from build123d import *

# Parameters (mm, degrees)
CROQUIS2_W              = 140
CROQUIS2_H              = 140
CROQUIS2_R              = 1.5
CROQUIS2_R_2            = 6
CROQUIS2_W_2            = 40
CROQUIS2_H_2            = 5
CROQUIS2_W_3            = 5
CROQUIS2_H_3            = 40
SALIENTE_EXTRUIR1_DEPTH = 5


with BuildPart() as part:
    # Croquis2 → Saliente-Extruir1 (new body)
    with BuildSketch(Plane(origin=(0, 0, 0), x_dir=(1, 0, 0), z_dir=(0, 1, 0))):
        with Locations((70, 70)):
            Rectangle(CROQUIS2_W, CROQUIS2_H)
        with Locations(Location((12.5, 107.5, 0), (0, 0, 270))):
            Circle(CROQUIS2_R, mode=Mode.SUBTRACT)
        with Locations(Location((12.5, 32.5, 0), (0, 0, 90))):
            Circle(CROQUIS2_R, mode=Mode.SUBTRACT)
        with Locations(Location((127.5, 32.5, 0), (0, 0, 270))):
            Circle(CROQUIS2_R, mode=Mode.SUBTRACT)
        with Locations(Location((127.5, 107.5, 0), (0, 0, 90))):
            Circle(CROQUIS2_R, mode=Mode.SUBTRACT)
        with Locations(Location((85.5, 37, 0), (0, 0, 270))):
            Circle(CROQUIS2_R, mode=Mode.SUBTRACT)
        with Locations(Location((77.75, 23.576606241, 0), (0, 0, 270))):
            Circle(CROQUIS2_R, mode=Mode.SUBTRACT)
        with Locations(Location((62.25, 23.576606241, 0), (0, 0, 270))):
            Circle(CROQUIS2_R, mode=Mode.SUBTRACT)
        with Locations(Location((54.5, 37, 0), (0, 0, 270))):
            Circle(CROQUIS2_R, mode=Mode.SUBTRACT)
        with Locations(Location((62.25, 50.423393759, 0), (0, 0, 270))):
            Circle(CROQUIS2_R, mode=Mode.SUBTRACT)
        with Locations(Location((77.75, 50.423393759, 0), (0, 0, 270))):
            Circle(CROQUIS2_R, mode=Mode.SUBTRACT)
        with Locations(Location((70, 30, 0), (0, 0, 270))):
            Circle(CROQUIS2_R_2, mode=Mode.SUBTRACT)
        with Locations((70, 127.5)):
            Rectangle(CROQUIS2_W_2, CROQUIS2_H_2, mode=Mode.SUBTRACT)
        with Locations((70, 12.5)):
            Rectangle(CROQUIS2_W_2, CROQUIS2_H_2, mode=Mode.SUBTRACT)
        with Locations((127.5, 70)):
            Rectangle(CROQUIS2_W_3, CROQUIS2_H_3, mode=Mode.SUBTRACT)
        with Locations((12.5, 70)):
            Rectangle(CROQUIS2_W_3, CROQUIS2_H_3, mode=Mode.SUBTRACT)
    extrude(amount=SALIENTE_EXTRUIR1_DEPTH)


solid = part.part
Here's how the part is built. I have some questions about the finished solid (model axes, mm). A direction names the side the tool comes from. Coordinates: 2 decimals unless noted, no trailing zeros. Write each loop counter-clockwise with the first axis right and the second up, starting at its lowest first coordinate (ties: lowest second). Pieces come first, ordered by that corner, then holes.
Item 1: On a 3-axis mill with a long thin cutter (end or side, diameter ignored), from which of +Z, -Z, +X, -X, +Y, -Y can I reach the whole of each face in a straight line? I mean faces 1 (the flat face through (12, 2, -90)), 2 (the flat face through (69, 2, -140)). Say none if no direction works.
Item 2: If we mould it in two halves opening along X, with no side actions, what happens to faces 3 (the flat face through (69, 5, -71)), 4 (the flat face through (70, 2, -15)), 5 (the flat face through (0, 2, -69))? For each: +X half, -X half, draft (parallel to the pull), parting line (faces both ways), or undercut.
Item 3: I want a section at B-B on y = 2.5. Count the separate pieces of the cut face and the enclosed holes in it, and give its area (3 significant figures).
Item 4: I want a section at A-A on z = -73. Write out the boundary of the cut face in (x, y), and give its area (3 significant figures).
Item 5: If I drill on line 1 (X direction, y = 0.9, z = -89); line 2 (X direction, y = 2.75, z = -107.5); line 3 (Z direction, x = 127.5, y = 3.3), over which ranges is the centre line in solid material (lowest first)?
Findings below:
1. face 1: +Y, -Y
1. face 2: -Z, +X, -X, +Y, -Y
2. face 3: draft
2. face 4: undercut
2. face 5: -X half
3. separate pieces: 1
3. enclosed holes: 15
3. area: 18,600 mm2
4. outline: (0, 0) - (10, 0) - (10, 5) - (0, 5) - close; (15, 0) - (125, 0) - (125, 5) - (15, 5) - close; (130, 0) - (140, 0) - (140, 5) - (130, 5) - close
4. area: 650 mm2
5. line 1: x = 0 to 10, 15 to 125, 130 to 140
5. line 2: x = 0 to 11, 14 to 126, 129 to 140
5. line 3: z = -140 to -109, -106 to -90, -50 to -34, -31 to 0
